from build123d import *

# Parameters (mm, degrees)
F0_W     = 500
F0_H     = 500
F0_R     = 31.5
F1_DEPTH = 25
F2_W     = 34
F2_H     = 34
F3_DEPTH = 455
F4_W     = 34
F4_H     = 34
F5_DEPTH = 25
F6_DEPTH = 17
F7_D     = 6


with BuildPart() as f1:
    # F0 (on Top) → F1 (new body)
    with BuildSketch(Plane.XY):
        Rectangle(F0_W, F0_H)
        with Locations((-180, -180)):
            Circle(F0_R, mode=Mode.SUBTRACT)
        with Locations((180, -180)):
            Circle(F0_R, mode=Mode.SUBTRACT)
        with Locations((-180, 180)):
            Circle(F0_R, mode=Mode.SUBTRACT)
        with Locations((180, 180)):
            Circle(F0_R, mode=Mode.SUBTRACT)
        with Locations((-180, -180)):
            Circle(F0_R)
        with Locations((180, -180)):
            Circle(F0_R)
        with Locations((-180, 180)):
            Circle(F0_R)
        with Locations((180, 180)):
            Circle(F0_R)
    extrude(amount=F1_DEPTH)

    # F2 (on face) → F3 (join)
    with BuildSketch(Plane.XY.offset(25)):
        with Locations((-233, 233)):
            Rectangle(F2_W, F2_H)
        with Locations((233, 233)):
            Rectangle(F2_W, F2_H)
        with Locations((233, -233)):
            Rectangle(F2_W, F2_H)
        with Locations((-233, -233)):
            Rectangle(F2_W, F2_H)
    extrude(amount=F3_DEPTH)

    # F4 (on face) → F5 (join)
    with BuildSketch(Plane.XY.offset(480)):
        Polygon((-250, -250), (250, -250), (250, 250), (-216, 250), (-216, 216), (-250, 216), align=None)
        with Locations((-233, 233)):
            Rectangle(F4_W, F4_H)
    extrude(amount=F5_DEPTH)

    # F0 (on Top) → F6 (join)
    with BuildSketch(Plane.XY):
        with Locations((-180, -180)):
            Circle(F0_R)
        with Locations((-180, 180)):
            Circle(F0_R)
        with Locations((180, 180)):
            Circle(F0_R)
        with Locations((180, -180)):
            Circle(F0_R)
    extrude(amount=-F6_DEPTH)

    # F7 (through all)
    with Locations(Plane(origin=(0, 0, 0), x_dir=(1, 0, 0), z_dir=(0, 0, -1))):
        with Locations((-233, -233), (233, -233), (233, 233), (-233, 233)):
            Hole(F7_D / 2)


solid = f1.part
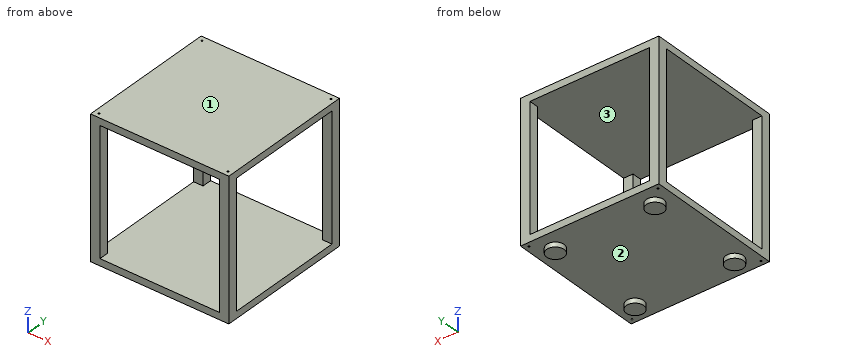
Check sheet for the modelled part. Datum: model origin and axes. Units: mm. Face numbers are marked on the shaded views. Give positions to 0.01 mm unless a question says otherwise; leave off trailing zeros. Loops run counter-clockwise (first coordinate to the right, second up) from the corner with the lowest first, then second, coordinate; pieces in that order, holes last. Notation, with made-up numbers: M 46.5,65.25 L 81.5,65.25 A21 cw 81.5,82.25 Z; hole C 41.25,-18.5 d2. An arc over 180 degrees is marked long. Use a Markdown table: item, result. Add a question column.
Q1. Sectioned sample at B-B, the plane x = -141. Record the cut outline in (y, z), then the cut area to 3 significant figures.
Q2. Scan lines: line 1 along Y through (x, z) = (233, 319.5); line 2 along Z through (x, y) = (-109.5, -25). Record each from-to range of solid material in increasing order. Write a range as [from, to].
Q3. Go/stop test with flat-tipped pins: pin 1 (5.5 mm diameter, centred on x = -233, y = -233, fed in from -Z); pin 2 (7 mm diameter, centred on x = 233, y = 233, fed in from -Z). Record where each tip stops, or that it passes through.
Q4. Mould release check, pull along Z, two halves, no side actions. Record for the marked faces 1, 2 and 3: pulls with the +Z half, pulls with the -Z half, needs draft (parallel to the pull), parting line crosses it, or undercut.
Q5. Sectioned sample at D-D, the plane y = 180. Record the cut outline in (x, z), then the cut area to 3 significant figures.
Q6. Sectioned sample at A-A, the plane z = 232. Record the cut outline in (x, y), then the cut area to 3 significant figures.
Verdict:
| question | item | result |
|---|---|---|
| 1 | outline | M -250,0 L 250,0 L 250,25 L -250,25 Z; M -250,480 L 250,480 L 250,505 L -250,505 Z |
| 1 | area | 25,000 mm^2 |
| 2 | line 1 | [-250, -236], [-230, -216], [216, 230], [236, 250] |
| 2 | line 2 | [0, 25], [480, 505] |
| 3 | pin 1 | through |
| 3 | pin 2 | z = 0 |
| 4 | face 1 | pulls with the +Z half |
| 4 | face 2 | pulls with the -Z half |
| 4 | face 3 | undercut |
| 5 | outline | M -250,0 L -211.5,0 L -211.5,-17 L -148.5,-17 L -148.5,0 L 148.5,0 L 148.5,-17 L 211.5,-17 L 211.5,0 L 250,0 L 250,25 L -250,25 Z; M -250,480 L 250,480 L 250,505 L -250,505 Z |
| 5 | area | 27,100 mm^2 |
| 6 | outline | M -250,-250 L -216,-250 L -216,-216 L -250,-216 Z; M -250,216 L -216,216 L -216,250 L -250,250 Z; M 216,-250 L 250,-250 L 250,-216 L 216,-216 Z; M 216,216 L 250,216 L 250,250 L 216,250 Z; hole C -233,-233 d6; hole C -233,233 d6; hole C 233,-233 d6; hole C 233,233 d6 |
| 6 | area | 4,510 mm^2 |
